```python
from build123d import *

# Parameters (mm, degrees)
SKETCH2_W           = 9.525
SKETCH2_H           = 25.4
BOSS_EXTRUDE1_DEPTH = 12.7
FILLET1_R           = 1.27
FILLET2_R           = 3.81
SKETCH15_R          = 3.981833791
CUT_EXTRUDE12_DEPTH = 55.150798834
SKETCH14_R          = 6.35
CUT_EXTRUDE13_DEPTH = 4.064
SKETCH17_R          = 1.778
CUT_EXTRUDE14_DEPTH = 56.155369014


with BuildPart() as part:
    # Sketch2 → Boss-Extrude1 (new body)
    with BuildSketch(Plane.XY):
        with Locations((9.39840893, -39.07155)):
            Rectangle(SKETCH2_W, SKETCH2_H)
    extrude(amount=BOSS_EXTRUDE1_DEPTH)

    # Fillet1
    fillet1_edges = [part.edges().sort_by_distance(p)[0] for p in [
        (4.63590893, -39.07155, 12.7),
        (14.16090893, -39.07155, 12.7),
        (4.63590893, -51.77155, 6.35),
        (4.63590893, -26.37155, 6.35),
        (14.16090893, -26.37155, 6.35),
        (14.16090893, -51.77155, 6.35),
    ]]
    fillet(fillet1_edges, radius=FILLET1_R)

    # Fillet2
    # the kernel refuses this fillet: 3.81 mm, written as the material it takes off along each edge
    with BuildSketch(Plane(origin=(14.16090893, -47.96155, 8.89), x_dir=(0, 0, 1), z_dir=(0, 1, 0))) as fillet2_piece_1:
        with BuildLine():
            CenterArc((2.54, -1.27), 1.27, 0, 90)
            Line((3.81, -1.27), (3.81, 0))
            Line((3.81, 0), (2.54, 0))
        make_face()
    revolve(axis=Axis((14.16090893, -47.96155, 8.89), (1, 0, 0)), revolution_arc=90, mode=Mode.SUBTRACT)
    with BuildSketch(Plane(origin=(14.16090893, -30.18155, 8.89), x_dir=(0, 1, 0), z_dir=(0, 0, -1))) as fillet2_piece_2:
        with BuildLine():
            CenterArc((2.54, -1.27), 1.27, 0, 90)
            Line((3.81, -1.27), (3.81, 0))
            Line((3.81, 0), (2.54, 0))
        make_face()
    revolve(axis=Axis((14.16090893, -30.18155, 8.89), (1, 0, 0)), revolution_arc=90, mode=Mode.SUBTRACT)
    with BuildSketch(Plane(origin=(4.63590893, -47.96155, 8.89), x_dir=(0, -1, 0), z_dir=(0, 0, -1))) as fillet2_piece_3:
        with BuildLine():
            CenterArc((2.54, -1.27), 1.27, 0, 90)
            Line((3.81, -1.27), (3.81, 0))
            Line((3.81, 0), (2.54, 0))
        make_face()
    revolve(axis=Axis((4.63590893, -47.96155, 8.89), (-1, 0, 0)), revolution_arc=90, mode=Mode.SUBTRACT)
    with BuildSketch(Plane(origin=(4.63590893, -30.18155, 8.89), x_dir=(0, 0, 1), z_dir=(0, -1, 0))) as fillet2_piece_4:
        with BuildLine():
            CenterArc((2.54, -1.27), 1.27, 0, 90)
            Line((3.81, -1.27), (3.81, 0))
            Line((3.81, 0), (2.54, 0))
        make_face()
    revolve(axis=Axis((4.63590893, -30.18155, 8.89), (-1, 0, 0)), revolution_arc=90, mode=Mode.SUBTRACT)
    with BuildSketch(Plane(origin=(14.16090893, -26.37155, 12.7), x_dir=(0, 0, -1), z_dir=(-1, 0, 0)), Plane(origin=(4.63590893, -51.77155, 12.7), x_dir=(0, 0, -1), z_dir=(1, 0, 0))) as fillet2_piece_5:
        with BuildLine():
            CenterArc((FILLET2_R, FILLET2_R), FILLET2_R, 180, 90)
            Line((0, FILLET2_R), (0, 0))
            Line((0, 0), (FILLET2_R, 0))
        make_face()
    extrude(amount=9.525, mode=Mode.SUBTRACT)

    # Sketch15 → Cut-Extrude12 (cut, through all)
    with BuildSketch(Plane.ZY.offset(-4.63590893)):
        with Locations((0, -39.07155)):
            Circle(SKETCH15_R)
    extrude(amount=-CUT_EXTRUDE12_DEPTH, mode=Mode.SUBTRACT)

    # Sketch14 → Cut-Extrude13 (cut)
    with BuildSketch(Plane.ZY.offset(-4.63590893)):
        with Locations((0, -39.07155)):
            Circle(SKETCH14_R)
    extrude(amount=-CUT_EXTRUDE13_DEPTH, mode=Mode.SUBTRACT)

    # Sketch17 → Cut-Extrude14 (cut, through all)
    with BuildSketch(Plane.XY.offset(12.7)):
        with Locations((9.39840893, -47.80915)):
            Circle(SKETCH17_R)
        with Locations((9.39840893, -30.33395)):
            Circle(SKETCH17_R)
    extrude(amount=-CUT_EXTRUDE14_DEPTH, mode=Mode.SUBTRACT)


solid = part.part
```
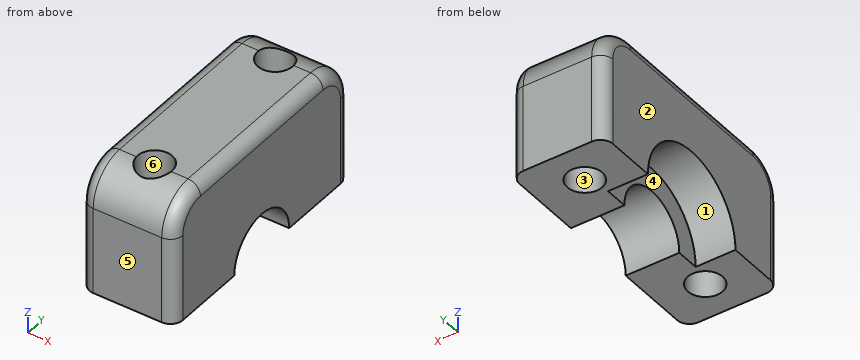
Design review of the part built by this model. Coordinates are the model's own, in mm. Face numbers are marked on the shaded views. A direction names the side the tool comes from. Coordinates: 2 decimals unless noted, no trailing zeros. Order: outer loops, then holes, each group sorted by start corner. A loop starts at its lowest first (then second) coordinate and runs counter-clockwise, first axis right, second up. Notation, with made-up numbers: M -14.75,80 L -6.75,80 A16 cw -6.75,106 Z; hole C 75,-29 d1. An arc over 180 degrees is marked long. Answer as a JSON object with one key per item and string values. Group by question number.
1) Tool access review of the marked faces 1 and 2: name each direction out of +Z, -Z, +X, -X, +Y, -Y from which nothing blocks a thin tool from reaching the whole face with its end or side.
2) Add section C-C, the plane y = -33. Write out the cut boundary in (x, z), then the cut area to 3 significant figures.
3) Add section B-B, the plane z = 8.5. Write out the cut boundary in (x, y), then the cut area to 3 significant figures.
4) Mouldability with a two-part tool opening along X and no side actions: class the marked faces 3, 4, 5 and 6 as pulls with the +X half, pulls with the -X half, needs draft (parallel to the pull), parting line crosses it, or undercut.
5) Wall thickness on L1, parallel to X at y = -30.25, z = 8.25; L2, parallel to X at y = -36, z = 4.75; L3, parallel to X at y = -40.25, z = 11.5: over which ranges is each line inside the solid? List them lowest first.
6) For pin 1 (5 mm diameter, centred on y = -40, z = 2, fed in from -X), flat-tipped, find the tip position at first contact; note if it passes through.
7) Add section A-A, the plane z = 2.75. Write out the cut boundary in (x, y).
8) Add section D-D, the plane z = 4.25. Write out the cut boundary in (x, y).
Computed values:
{
 "1": {"face 1": "-Z, -X", "face 2": "+Z, -Z, -X, +Y, -Y"},
 "2": {"outline": "M 4.64,1.86 L 8.7,1.86 L 8.7,0 L 14.16,0 L 14.16,11.43 A1.27 ccw 12.89,12.7 L 5.91,12.7 A1.27 ccw 4.64,11.43 Z", "area": "113 mm^2"},
 "3": {"outline": "M 4.64,-50.5 A1.27 ccw 5.91,-51.77 L 12.89,-51.77 A1.27 ccw 14.16,-50.5 L 14.16,-27.64 A1.27 ccw 12.89,-26.37 L 5.91,-26.37 A1.27 ccw 4.64,-27.64 Z; hole C 9.4,-47.81 d3.56; hole C 9.4,-30.33 d3.56", "area": "221 mm^2"},
 "4": {"face 3": "undercut", "face 4": "pulls with the -X half", "face 5": "needs draft", "face 6": "undercut"},
 "5": {"L1": "x = 4.64 to 7.62, 11.17 to 14.16", "L2": "x = 8.7 to 14.16", "L3": "x = 4.64 to 14.16"},
 "6": {"pin 1": "stops at x = 8.7"},
 "7": {"outline": "M 4.64,-50.5 A1.27 ccw 5.91,-51.77 L 12.89,-51.77 A1.27 ccw 14.16,-50.5 L 14.16,-41.95 L 8.7,-41.95 L 8.7,-44.8 L 4.64,-44.8 Z; M 4.64,-33.35 L 8.7,-33.35 L 8.7,-36.19 L 14.16,-36.19 L 14.16,-27.64 A1.27 ccw 12.89,-26.37 L 5.91,-26.37 A1.27 ccw 4.64,-27.64 Z; hole C 9.4,-47.81 d3.56; hole C 9.4,-30.33 d3.56"},
 "8": {"outline": "M 4.64,-50.5 A1.27 ccw 5.91,-51.77 L 12.89,-51.77 A1.27 ccw 14.16,-50.5 L 14.16,-27.64 A1.27 ccw 12.89,-26.37 L 5.91,-26.37 A1.27 ccw 4.64,-27.64 L 4.64,-34.35 L 8.7,-34.35 L 8.7,-43.79 L 4.64,-43.79 Z; hole C 9.4,-47.81 d3.56; hole C 9.4,-30.33 d3.56"}
}
